Check sheet for the modelled part. Datum: model origin and axes. Units: mm. Face numbers are marked on the shaded views. Round coordinates to 2 decimals unless told otherwise and drop trailing zeros. Order: outer loops, then holes, each group sorted by start corner. A loop starts at its lowest first (then second) coordinate and runs counter-clockwise, first axis right, second up.
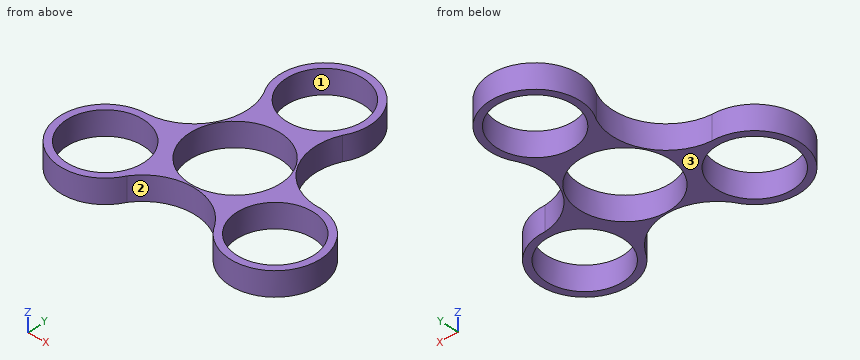
```python
from build123d import *

# Parameters (mm, degrees)
F0_R     = 11.2
F0_R_2   = 13.2
F1_DEPTH = 7


with BuildPart() as f1:
    # F0 (on Top) → F1 (new body)
    with BuildSketch(Plane.XY):
        with BuildLine():
            ThreePointArc((23.78745, -0.927916), (11.678462, 6.964523), (11.307953, 21.413775))
            ThreePointArc((11.307953, 21.413775), (-0.205819, 41.421737), (-11.090126, 21.064494))
            ThreePointArc((-11.090126, 21.064494), (-11.870685, 6.631583), (-24.19885, -0.913913))
            ThreePointArc((-24.19885, -0.913913), (-35.769367, -20.889113), (-12.697324, -20.136578))
            ThreePointArc((-12.697324, -20.136578), (0.192223, -13.596106), (12.890897, -20.499863))
            ThreePointArc((12.890897, -20.499863), (35.975186, -20.532624), (23.78745, -0.927916))
        make_face()
        with Locations((-24.442131, -14.111671)):
            Circle(F0_R, mode=Mode.SUBTRACT)
        with Locations((24.442131, -14.111671)):
            Circle(F0_R, mode=Mode.SUBTRACT)
        Circle(F0_R_2, mode=Mode.SUBTRACT)
        with Locations((0, 28.223341)):
            Circle(F0_R, mode=Mode.SUBTRACT)
    extrude(amount=F1_DEPTH)


solid = f1.part
```
Item 1: Sectioned sample at C-C (x = 0). Record the cut outline in (y, z), and give its area (3 significant figures).
Answer:
outline: (-13.59, 0) - (-13.2, 0) - (-13.2, 7) - (-13.59, 7) - close; (13.2, 0) - (17.02, 0) - (17.02, 7) - (13.2, 7) - close; (39.42, 0) - (41.42, 0) - (41.42, 7) - (39.42, 7) - close
area: 43.5 mm2
Item 2: Scan lines: line 1 along X through (y, z) = (-23.5, 2.5); line 2 along X through (y, z) = (-21.5, 5); line 3 along Y through (x, z) = (-9, 2). Record each from-to range of solid material in increasing order.
Answer:
line 1: x = -33.72 to -30.55, -18.33 to -15.16, 15.16 to 18.33, 30.55 to 33.72
line 2: x = -35.38 to -32.86, -16.02 to -13.5, 13.5 to 16.02, 32.86 to 35.38
line 3: y = -16.45 to -9.66, 9.66 to 21.56, 34.89 to 37.88
Item 3: Sectioned sample at D-D (y = 20). Record the cut outline in (x, z), and give its area (3 significant figures).
Answer:
outline: (-10.65, 0) - (-7.6, 0) - (-7.6, 7) - (-10.65, 7) - close; (7.6, 0) - (10.7, 0) - (10.7, 7) - (7.6, 7) - close
area: 43.0 mm2
Item 4: Go/stop test with flat-tipped pins: P1, Ø1.5, axis at x = -26.5, z = 3.5, coming from the -Y side; P2, Ø1, axis at x = 10.5, z = 3.5, coming from the -Y side; P3, Ø18, axis at x = 0, y = 28.22, coming from the +Z side; P4, Ø1, axis at x = -7, z = 3, coming from the +Y side. Record where each tip stops, or that it passes through.
Answer:
P1: stops at y = -27.25
P2: stops at y = -18.19
P3: passes through
P4: stops at y = 39.71
Item 5: Release check for a two-part mould opening along Y. For the marked faces 1, 2 and 3 record: released by +Y, released by -Y, zero draft, split by the parting line, or undercut.
Answer:
face 1: undercut
face 2: released by -Y
face 3: zero draft
Item 6: Sectioned sample at B-B (z = 5.75). Record the cut outline in (x, y), and give its area (3 significant figures).
Answer:
outline: (-24.2, -0.91) arc R13.2 ccw (long way) to (-12.7, -20.14) arc R15.54 cw to (12.89, -20.5) arc R13.2 ccw (long way) to (23.79, -0.93) arc R15.54 cw to (11.31, 21.41) arc R13.2 ccw (long way) to (-11.09, 21.06) arc R15.54 cw to start; hole circle Ø22.4 at (-24.44, -14.11); hole circle Ø26.4 at (0, 0); hole circle Ø22.4 at (0, 28.22); hole circle Ø22.4 at (24.44, -14.11)
area: 749 mm2
Item 7: Sectioned sample at A-A (y = 31). Record the cut outline in (x, z).
Answer:
outline: (-12.9, 0) - (-10.85, 0) - (-10.85, 7) - (-12.9, 7) - close; (10.85, 0) - (12.9, 0) - (12.9, 7) - (10.85, 7) - close
